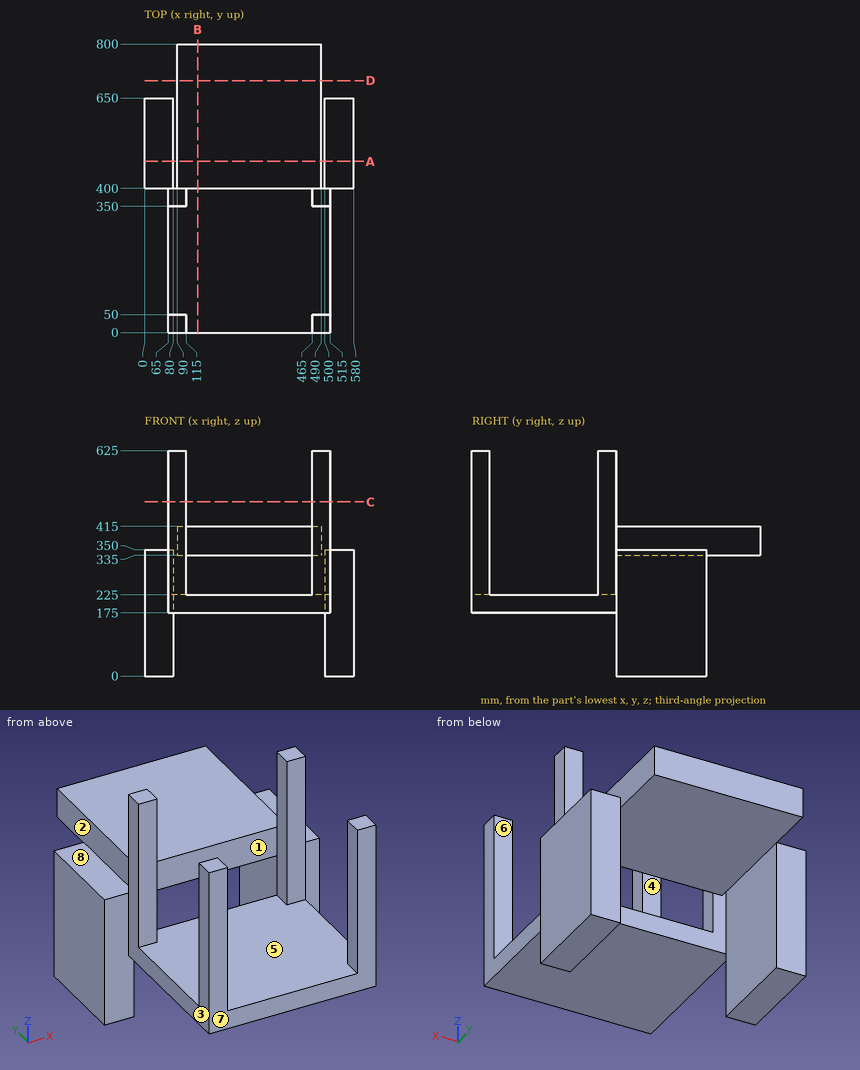
Geometry check sheet. Reference: drawing and pictorial views, mm from the part's lowest x, y, z. A direction names the side the tool comes from. Round coordinates to 2 decimals unless told otherwise and drop trailing zeros. Order: outer loops, then holes, each group sorted by start corner. A loop starts at its lowest first (then second) coordinate and runs counter-clockwise, first axis right, second up. Notation, with made-up numbers: M 47.5,-30.75 L 84.5,-30.75 A20 cw 84.5,-17.75 Z; hole C -31.5,-1.75 d7. An arc over 180 degrees is marked long. One line per item, written item: value. Start each with the question number.
1. Section check C-C on z = 483. Enter the section's corners in (x, y).
2. Section check B-B on x = 147. Enter the section's corners in (y, z).
3. Access from +Z, -Z, +X, -X, +Y, -Y to the whole of each face (thin tool, end or side, straight path). Record for the marked faces 1, 2, 3 and 4.
4. Scan lines: line 1 along Y through (x, z) = (489.5, 578.5); line 2 along X through (y, z) = (507, 27.5); line 3 along Y through (x, z) = (78.5, 124.5). Record each from-to range of solid material in increasing order.
5. Section check D-D on y = 698.5. Enter the section's corners in (x, z), and give its area (3 significant figures).
6. Section check A-A on y = 474.5. Enter the section's corners in (x, z), and give its area (3 significant figures).
7. Gauge pin test, flat ends, axial feed: P1, Ø15, axis at y = 379.5, z = 357, coming from the +X side; P2, Ø15, axis at x = 490.5, z = 489.5, coming from the +Y side; P3, Ø2, axis at x = 411, y = 214, coming from the -Z side. Record the tip position at first contact, or that the pin passes through.
8. Release check for a two-part mould opening along Y. For the marked faces 5, 6, 7 and 8 record: released by +Y, released by -Y, zero draft, split by the parting line, or undercut.
Results found:
1. outline: M 65,0 L 115,0 L 115,50 L 65,50 Z; M 65,350 L 115,350 L 115,400 L 65,400 Z; M 465,0 L 515,0 L 515,50 L 465,50 Z; M 465,350 L 515,350 L 515,400 L 465,400 Z
2. outline: M 0,175 L 400,175 L 400,225 L 0,225 Z; M 400,335 L 800,335 L 800,415 L 400,415 Z
3. face 1: +Z, -Y
3. face 2: +Z, -Z, +Y
3. face 3: +Z, -Z, -X, -Y
3. face 4: +Z, +X, -X
4. line 1: 0 to 50, 350 to 400
4. line 2: 0 to 80, 500 to 580
4. line 3: 400 to 650
5. outline: M 90,335 L 490,335 L 490,415 L 90,415 Z
5. area: 32,000 mm^2
6. outline: M 0,0 L 80,0 L 80,350 L 0,350 Z; M 90,335 L 490,335 L 490,415 L 90,415 Z; M 500,0 L 580,0 L 580,350 L 500,350 Z
6. area: 88,000 mm^2
7. P1: x = 515
7. P2: y = 400
7. P3: z = 175
8. face 5: undercut
8. face 6: undercut
8. face 7: released by -Y
8. face 8: zero draft
